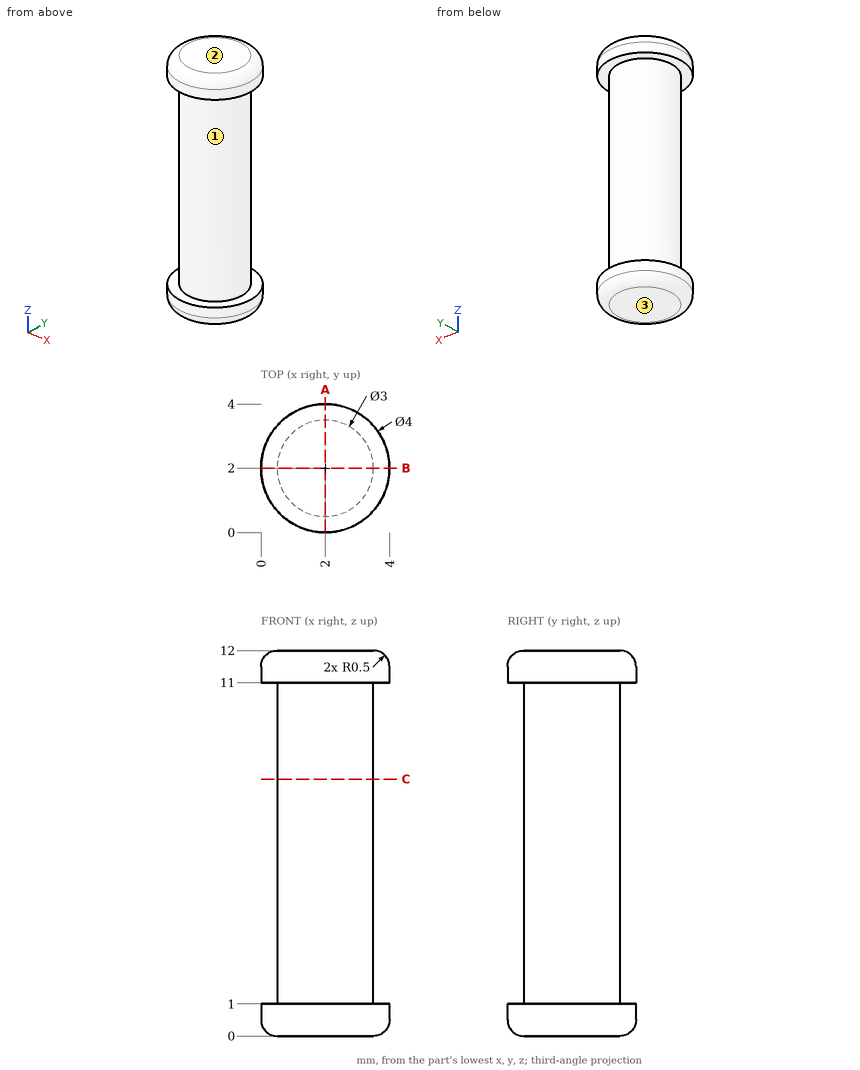
For this review, use the dimensioned drawing (mm, ordinates from the lowest corner) and the shaded views. Give positions to 0.01 mm unless a question says otherwise; leave off trailing zeros. Write each loop counter-clockwise with the first axis right and the second up, starting at its lowest first coordinate (ties: lowest second). Pieces come first, ordered by that corner, then holes. Notation, with made-up numbers: M -21.75,46.5 L -6.75,46.5 A20 cw -6.75,58.5 Z; hole C 83.25,65.25 d6. An arc over 180 degrees is marked long. Answer as a JSON object with one key per item and string values. Group by question number.
1) For line 1 along Z through (x, y) = (0.5, 1.65); line 2 along Y through (x, z) = (2, 7.5); line 3 along Z through (x, y) = (3.05, 3.6), list the stretches that pass through material, from the lowest coordinate up.
2) Mouldability with a two-part tool opening along Z and no side actions: class the marked faces 1, 2 and 3 as released by +Z, released by -Z, zero draft, split by the parting line, or undercut.
3) Clearance check with a flat-ended pin moving along its axis: pin 1 Ø1 at (y, z) = (2.5, 5.5) entering from +X. State where the tip first meets the part, or that it passes through.
4) We need section A-A (x = 2). Give the boundary of the cut face in (y, z).
5) We need section C-C (z = 8). Give the boundary of the cut face in (x, y), and give its area (3 significant figures).
Answer key:
{
 "1": {"line 1": "z = 0 to 1, 11 to 12", "line 2": "y = 0.5 to 3.5", "line 3": "z = 0.22 to 1, 11 to 11.78"},
 "2": {"face 1": "undercut", "face 2": "released by +Z", "face 3": "released by -Z"},
 "3": {"pin 1": "stops at x = 3.5"},
 "4": {"outline": "M 0,0.5 A0.5 ccw 0.5,0 L 3.5,0 A0.5 ccw 4,0.5 L 4,1 L 3.5,1 L 3.5,11 L 4,11 L 4,11.5 A0.5 ccw 3.5,12 L 0.5,12 A0.5 ccw 0,11.5 L 0,11 L 0.5,11 L 0.5,1 L 0,1 Z"},
 "5": {"outline": "C 2,2 d3", "area": "7.07 mm²"}
}
